The drawing under review shows one solid part. Ordinate dimensions are in mm from its lowest x, y, z. Give positions to 0.01 mm unless a question says otherwise; leave off trailing zeros. Loops run counter-clockwise (first coordinate to the right, second up) from the corner with the lowest first, then second, coordinate; pieces in that order, holes last. Notation, with made-up numbers: (71, 0) - (97, 0) arc R21 ccw to (97, 25) - close; hole circle Ø6 at (-39.5, 0.5). An arc over 180 degrees is marked (long way). Write each question's results on one line, items separated by ' | '.
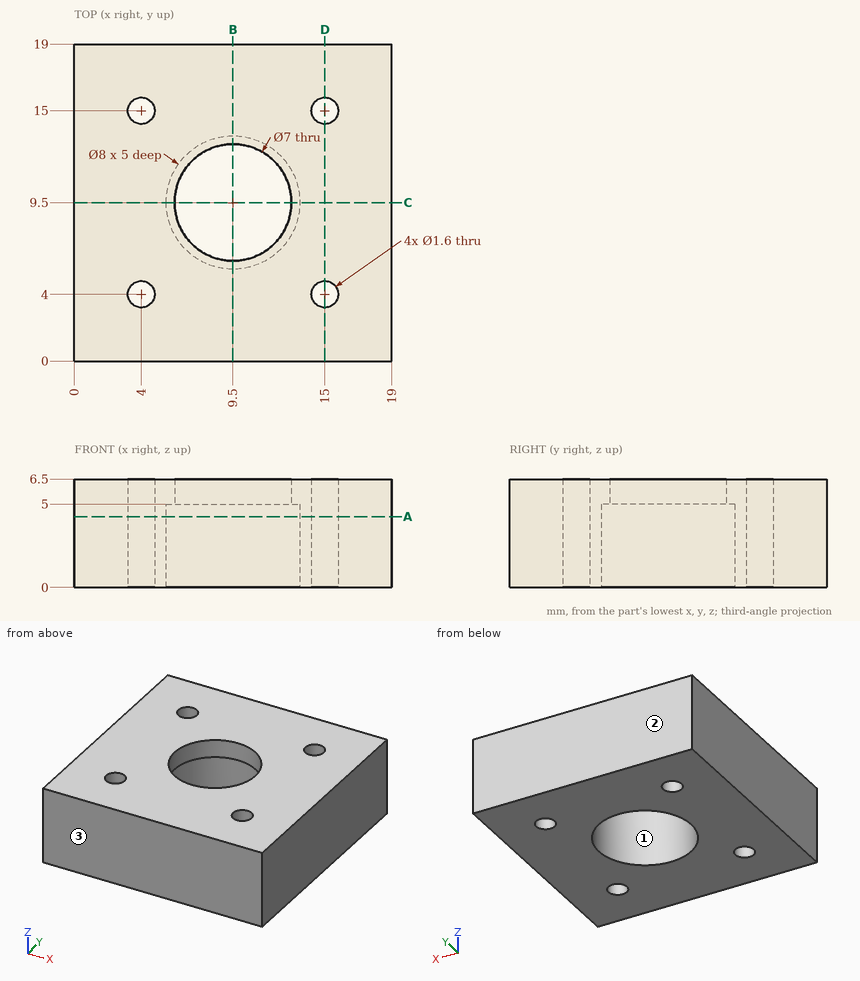
(1) Take a section at B-B on x = 9.5. Give the boundary of the cut face in (y, z).
Answers below:
outline: (0, 0) - (5.5, 0) - (5.5, 5) - (6, 5) - (6, 6.5) - (0, 6.5) - close; (13, 5) - (13.5, 5) - (13.5, 0) - (19, 0) - (19, 6.5) - (13, 6.5) - close
(2) Take a section at D-D on x = 15. Give the boundary of the cut face in (y, z).
Answers below:
outline: (0, 0) - (3.2, 0) - (3.2, 6.5) - (0, 6.5) - close; (4.8, 0) - (14.2, 0) - (14.2, 6.5) - (4.8, 6.5) - close; (15.8, 0) - (19, 0) - (19, 6.5) - (15.8, 6.5) - close
(3) Insertion check: P1, Ø4, axis at x = 9, y = 11, coming from the -Z side. The pin has a flat end and moves straight along its axis. Give the tip position at first contact, or say it passes through.
Answers below:
P1: z = 5
(4) Wall thickness on line 1 along Y through (x, z) = (15, 2.5); line 2 along Y through (x, z) = (9.5, 2.4); line 3 along X through (y, z) = (14.75, 4): over which ranges is each line inside the solid? List them lowest first. Write a range as from..to.
Answers below:
line 1: 0..3.2, 4.8..14.2, 15.8..19 | line 2: 0..5.5, 13.5..19 | line 3: 0..3.24, 4.76..14.24, 15.76..19
(5) Draft analysis for pull direction Y (two halves, no side actions). For the marked faces 1, 2 and 3, state which applies: pulls with the +Y half, pulls with the -Y half, needs draft (parallel to the pull), parting line crosses it, or undercut.
Answers below:
face 1: undercut | face 2: pulls with the +Y half | face 3: pulls with the -Y half
(6) Take a section at A-A on z = 4.25. Give the boundary of the cut face in (x, y).
Answers below:
outline: (0, 0) - (19, 0) - (19, 19) - (0, 19) - close; hole circle Ø1.6 at (4, 4); hole circle Ø1.6 at (4, 15); hole circle Ø8 at (9.5, 9.5); hole circle Ø1.6 at (15, 4); hole circle Ø1.6 at (15, 15)
